Geometry check sheet. Reference: the model listing, model coordinates, mm. A direction names the side the tool comes from. Round coordinates to 2 decimals unless told otherwise and drop trailing zeros. Write each loop counter-clockwise with the first axis right and the second up, starting at its lowest first coordinate (ties: lowest second). Pieces come first, ordered by that corner, then holes. Notation, with made-up numbers: M 14,-38 L 35,-38 A14 ccw 35,-11 Z; hole C 76,-39.75 d10. An arc over 180 degrees is marked long. Put each result on its own line as item: value. Start each with the question number.
(1) Section check B-B on z = 7.5. Record the cut outline in (x, y).
(2) Section check A-A on y = 72.5. Record the cut outline in (x, z).
(3) Section check D-D on y = 235.5. Record the cut outline in (x, z).
(4) Section check C-C on x = 55.5. Record the cut outline in (y, z), then the cut area to 3 significant figures.
(5) Tool access check on faces 1 (the flat face through (60.039, 224, 0)), 2 (the cylindrical face through (9.751, 103.008, -13.028)). Record the directions out of +Z, -Z, +X, -X, +Y, -Y that give a thin tool (end or side, any length) a straight path to the whole face; none if there is none.
(6) Mould release check, pull along X, two halves, no side actions. Record for faces 3 (the cylindrical face through (21.588, 141.216, -13.028)), 4 (the flat face through (21, 124, -11)), 5 (the flat face through (4.234, 142.595, -13.028)), 6 (the flat face through (23.13, 11.71, -13.03)): pulls with the +X half, pulls with the -X half, needs draft (parallel to the pull), parting line crosses it, or undercut.
(7) Gauge pin test, flat ends, axial feed: pin 1 (2 mm diameter, centred on y = 72.5, z = 13, fed in from +X); pin 2 (5 mm diameter, centred on x = -8, z = 0.5, fed in from -Y); pin 3 (11 mm diameter, centred on y = 219.5, z = -1.5, fed in from -X). Record the tip position at first contact, or that the pin passes through.
(8) Material ranges on probe 1 along Z at (x, y) = (58.5, 243); probe 2 along Y at (x, z) = (5, -1); probe 3 along Y at (x, z) = (47, -11.25), recorded low to high.
from build123d import *

# Parameters (mm, degrees)
BOSS_EXTRUDE1_START = 11
SKETCH2_R           = 12.7
SKETCH2_R_2         = 8
SKETCH2_R_3         = 15
BOSS_EXTRUDE1_DEPTH = 4
LPATTERN1_COUNT     = 2
LPATTERN1_PITCH     = 26
BOSS_EXTRUDE2_DEPTH = 15
SKETCH4_R           = 12.7
SKETCH4_R_2         = 11
SKETCH4_R_3         = 15
SKETCH4_R_4         = 13
BOSS_EXTRUDE3_DEPTH = 15
CHAMFER2_SIZE       = 0.5


with BuildPart() as part:
    # Sketch2 → Boss-Extrude1 (new body)
    with BuildSketch(Plane.XY.offset(BOSS_EXTRUDE1_START)):
        with BuildLine():
            Line((30.078103468, 30.102899094), (30.078103468, 104.858637586))
            Line((30.078103468, 104.858637586), (43.656234688, 145.478166756))
            Line((43.656234688, 145.478166756), (60.038536544, 194.486485935))
            Line((60.038536544, 194.486485935), (60.038536544, 254.427096014))
            ThreePointArc((60.038536544, 254.427096014), (45.05832001, 260.632104877), (30.078103469, 254.427096029))
            Line((30.078103469, 254.427096029), (22.62926434, 194.486485916))
            Line((22.62926434, 194.486485916), (-14.683335653, 89.230795609))
            Line((-14.683335653, 89.230795609), (-17.49123357, 0.553848547))
            ThreePointArc((-17.49123357, 0.553848547), (-3.415184823, -17.163522734), (16.370945819, -6.184022397))
            Line((16.370945819, -6.184022397), (30.078103468, 30.102899094))
        make_face()
        Circle(SKETCH2_R, mode=Mode.SUBTRACT)
        with Locations((45.058319997, 232.788133995)):
            Circle(SKETCH2_R_2, mode=Mode.SUBTRACT)
        with Locations((42.85515341, 200.574247039)):
            Circle(SKETCH2_R_2, mode=Mode.SUBTRACT)
        with Locations((32.877400798, 166.36480954)):
            Circle(SKETCH2_R_2, mode=Mode.SUBTRACT)
        with Locations((22.629264347, 133.284451418)):
            Circle(SKETCH2_R_2, mode=Mode.SUBTRACT)
        with Locations((10.792452444, 95.075946031)):
            Circle(SKETCH2_R_2, mode=Mode.SUBTRACT)
        with Locations((5.075535148, 44.712849864)):
            Circle(SKETCH2_R_3, mode=Mode.SUBTRACT)
    extrude(amount=BOSS_EXTRUDE1_DEPTH)


with BuildPart() as lpattern1_1:
    # LPattern1: pattern copy
    add(part.part.moved(Location(Vector(0, 0, -1) * (1 * LPATTERN1_PITCH))))


with BuildPart() as part_1:
    add(part.part)

    add(lpattern1_1.part)  # Boss-Extrude2 merges LPattern1_1
    # Sketch3 → Boss-Extrude2 (add, symmetric)
    with BuildSketch(Plane.XY):
        Polygon((60.038536544, 194.486485935), (60.038536544, 254.427096014), (64.038536544, 254.427096014), (64.038536544, 193.835634299), (48.186924823, 146.414896158), (44.393265771, 147.683025095), align=None)
    extrude(amount=BOSS_EXTRUDE2_DEPTH, both=True)

    # Sketch4 → Boss-Extrude3 (add, symmetric)
    # profile 1 of 2: a face of its own
    with BuildSketch(Plane.XY):
        Circle(SKETCH4_R)
        Circle(SKETCH4_R_2, mode=Mode.SUBTRACT)
    # profile 2 of 2: a face of its own
    with BuildSketch(Plane.XY):
        with Locations((5.075535148, 44.712849864)):
            Circle(SKETCH4_R_3)
        with Locations((5.075535148, 44.712849864)):
            Circle(SKETCH4_R_4, mode=Mode.SUBTRACT)
    extrude(amount=BOSS_EXTRUDE3_DEPTH, both=True)

    # Chamfer2
    chamfer2_edges = [part_1.edges().sort_by_distance(p)[0] for p in [
        (-11, 0, -15),
        (-11, 0, 15),
        (-7.924464852, 44.712849864, -15),
        (-7.924464852, 44.712849864, 15),
    ]]
    chamfer(chamfer2_edges, length=CHAMFER2_SIZE)


solid = part_1.part
Answers follow:
1. outline: C 0,0 d25.4; C 5.08,44.71 d30; M 44.39,147.68 L 48.19,146.41 L 64.04,193.84 L 64.04,254.43 L 60.04,254.43 L 60.04,194.49 Z; hole C 0,0 d22; hole C 5.08,44.71 d26
2. outline: M -15.21,-15 L 30.08,-15 L 30.08,-11 L -15.21,-11 Z; M -15.21,11 L 30.08,11 L 30.08,15 L -15.21,15 Z
3. outline: M 27.73,-15 L 37.53,-15 L 37.53,-11 L 27.73,-11 Z; M 27.73,11 L 37.53,11 L 37.53,15 L 27.73,15 Z; M 52.58,-15 L 64.04,-15 L 64.04,15 L 52.58,15 L 52.58,11 L 60.04,11 L 60.04,-11 L 52.58,-11 Z
4. outline: M 168.29,-15 L 257.88,-15 L 257.88,-11 L 180.91,-11 L 180.91,11 L 257.88,11 L 257.88,15 L 168.29,15 Z
4. area: 994 mm^2
5. face 1: -X, +Y
5. face 2: +Z, -Z
6. face 3: undercut
6. face 4: needs draft
6. face 5: pulls with the -X half
6. face 6: pulls with the +X half
7. pin 1: stops at x = 30.08
7. pin 2: stops at y = -11.45
7. pin 3: stops at x = 60.04
8. probe 1: z = -15 to -11, 11 to 15
8. probe 2: y = -11.67 to -9.8, 9.8 to 11.67, 29.71 to 31.71, 57.71 to 59.71
8. probe 3: y = 146.81 to 193.73, 207.42 to 225.03, 240.55 to 260.54
